Answer from the drawing. Dimensions are ordinates in mm from the lowest x, y and z of the part. A direction names the side the tool comes from. Give positions to 0.01 mm unless a question says otherwise; leave off trailing zeros. Loops run counter-clockwise (first coordinate to the right, second up) from the corner with the lowest first, then second, coordinate; pieces in that order, holes last. Notation, with made-up numbers: (58.5, -9.75) -> (114.5, -9.75) arc R32 cw to (114.5, 16.25) -> close; hole circle Ø7 at (-3, 25.5). An arc over 180 degrees is marked (long way). Write each question's results on one line, items separated by ' | '. Start each with the question number.
Item 1: Section C-C on z = 4 is taken. Write down the section's boundary in (x, y).
Item 2: Which of the six approach directions +Z, -Z, +X, -X, +Y, -Y give full straight-line access (tool end or side, diameter ignored) to the marked faces 5 and 6?
Item 3: Each of these flat-tipped pins is pushed along its axis until it touches: P1, Ø2, axis at x = 2.89, z = 2.5, coming from the -Y side; P2, Ø3, axis at y = 6, z = 2, coming from the -X side. Where does it stop, or does it pass through?
Item 4: Section B-B on y = 8.75 is taken. Write down the section's boundary in (x, z).
Item 5: Section D-D on y = 11.25 is taken. Write down the section's boundary in (x, z).
Item 6: Find the intervals of material crossed by line 1 (Y direction, x = 1.95, z = 1.4); line 2 (X direction, y = 1, z = 2.4) (1 decimal); line 3 (Z direction, x = 2.8, y = 14.25), in increasing order.
Item 7: Section A-A on y = 7 is taken. Write down the section's boundary in (x, z).
Item 8: Determine the mould class of the marked faces 1, 2, 3 and 4 for opening direction Z: +Z half, -Z half, draft (parallel to the pull), parting line (faces both ways), or undercut.
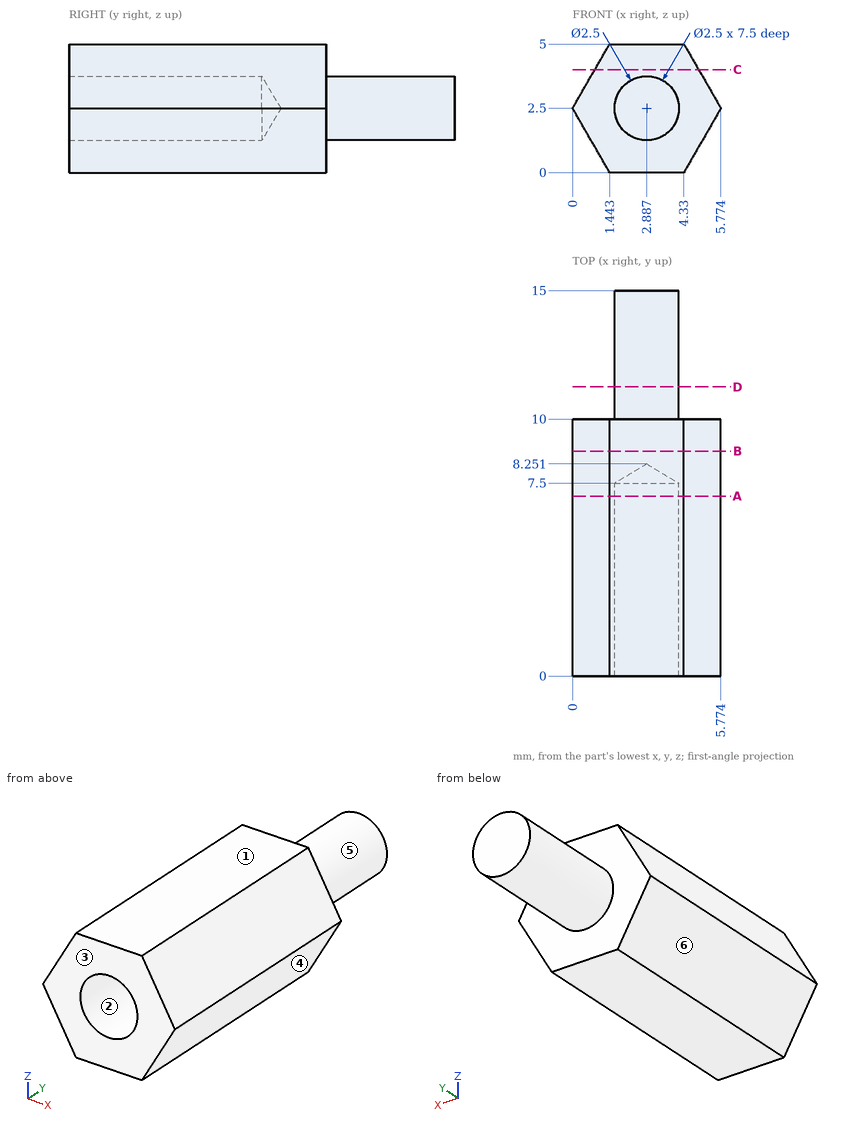
Findings:
1) outline: (0.87, 0) -> (4.91, 0) -> (4.91, 10) -> (0.87, 10) -> close
2) face 5: +Y | face 6: -Z, -X, +Y, -Y
3) P1: y = 7.65 | P2: x = 0
4) outline: (0, 2.5) -> (1.44, 0) -> (4.33, 0) -> (5.77, 2.5) -> (4.33, 5) -> (1.44, 5) -> close
5) outline: circle Ø2.5 at (2.89, 2.5)
6) line 1: 0 to 10 | line 2: 0.1 to 1.6, 4.1 to 5.7 | line 3: 1.25 to 3.75
7) outline: (0, 2.5) -> (1.44, 0) -> (4.33, 0) -> (5.77, 2.5) -> (4.33, 5) -> (1.44, 5) -> close; hole circle Ø2.5 at (2.89, 2.5)
8) face 1: +Z half | face 2: undercut | face 3: draft | face 4: -Z half
